```python
from build123d import *

# Parameters (mm, degrees)
SZKIC1_W                         = 100
SZKIC1_H                         = 28
OGOLNY_KSZTALT_DEPTH             = 50
ZAKRZYWUIENIE_OUTSIDE_W          = 53.052
ZAKRZYWUIENIE_OUTSIDE_H          = 75.052
WYCIECIE_KSZTAL_PRZOD_DEPTH      = 105
WYCIECIE_KSZTALTU_TYL_DEPTH      = 23
WYCIECIE_KSZTALTU_TYL_DEPTH_BACK = 99.5
SZKIC4_W                         = 30.5
SZKIC4_H                         = 10
SZKIC5_W                         = 39
SZKIC5_H                         = 10
PODBICIE_TYL_SPOD_DEPTH          = 5.5
SZKIC6_W                         = 100
SZKIC6_H                         = 8
PODBICIE_SRODEK_SPOD_DEPTH       = 4
PRZYCIECIE_OD_GORY_DEPTH         = 40
OTWORY_NA_SRUBY_DEPTH            = 90
OTWORY_NA_SRUBY_DEPTH_BACK       = 71
SZKIC8_R                         = 1.25
SZKIC9_W                         = 9
SZKIC9_H                         = 10
KTIR_KABLE_DEPTH                 = 10
WYTNIJ_WYCI_GNI_CIE3_DEPTH       = 84
WYTNIJ_WYCI_GNI_CIE3_DEPTH_BACK  = 81
SZKIC10_W                        = 29
SZKIC10_H                        = 10
WYTNIJ_WYCI_GNI_CIE4_DEPTH       = 59
WYTNIJ_WYCI_GNI_CIE4_DEPTH_BACK  = 55
SZKIC11_W                        = 10
SZKIC11_H                        = 15
SZKIC11_W_2                      = 17


with BuildPart() as part:
    # Szkic1 → ogolny ksztalt (new body)
    with BuildSketch(Plane(origin=(0, 0, 0), x_dir=(1, 0, 0), z_dir=(0, 1, 0))):
        with Locations((-50, 14)):
            Rectangle(SZKIC1_W, SZKIC1_H)
    extrude(amount=OGOLNY_KSZTALT_DEPTH)

    # zakrzywuienie outside → wyciecie ksztal przod (cut)
    with BuildSketch(Plane(origin=(0, 0, 0), x_dir=(0, 0, -1), z_dir=(1, 0, 0))):
        with Locations((14, 25)):
            Rectangle(ZAKRZYWUIENIE_OUTSIDE_W, ZAKRZYWUIENIE_OUTSIDE_H)
        with BuildLine():
            Line((28, 0), (18, 0))
            Line((18, 0), (0, 0))
            Line((0, 0), (0, 50))
            Line((0, 50), (18, 50))
            add(Edge.make_bspline(
                [(18, 50), (14.693585387, 12.992576306), (20.397077092, 0.692779903), (28, 0)],
                knots=[0, 0, 0, 0, 1, 1, 1, 1], degree=3))
        make_face(mode=Mode.SUBTRACT)
    extrude(amount=-WYCIECIE_KSZTAL_PRZOD_DEPTH, mode=Mode.SUBTRACT)

    # Szkic4 → wyciecie ksztaltu tyl (cut, two sides: drawn at the far end of the back side and taken through both)
    with BuildSketch(Plane(origin=(0, 0, 0), x_dir=(-1, 0, 0), z_dir=(0, -1, 0)).offset(-WYCIECIE_KSZTALTU_TYL_DEPTH_BACK)):
        with Locations((84.75, 5)):
            Rectangle(SZKIC4_W, SZKIC4_H)
        with Locations((15.25, 5)):
            Rectangle(SZKIC4_W, SZKIC4_H)
    extrude(amount=WYCIECIE_KSZTALTU_TYL_DEPTH + WYCIECIE_KSZTALTU_TYL_DEPTH_BACK, mode=Mode.SUBTRACT)

    # Szkic5 → podbicie tyl(spod) (cut)
    with BuildSketch(Plane(origin=(0, 0, 0), x_dir=(-1, 0, 0), z_dir=(0, -1, 0))):
        with Locations((50, 5)):
            Rectangle(SZKIC5_W, SZKIC5_H)
    extrude(amount=-PODBICIE_TYL_SPOD_DEPTH, mode=Mode.SUBTRACT)

    # Szkic6 → podbicie srodek(spod) (cut)
    with BuildSketch(Plane(origin=(0, 0, 0), x_dir=(-1, 0, 0), z_dir=(0, -1, 0))):
        with Locations((50, 14)):
            Rectangle(SZKIC6_W, SZKIC6_H)
    extrude(amount=-PODBICIE_SRODEK_SPOD_DEPTH, mode=Mode.SUBTRACT)

    # Szkic7 → przyciecie od gory (cut)
    with BuildSketch(Plane(origin=(0, 50, 0), x_dir=(1, 0, 0), z_dir=(0, 1, 0))):
        Polygon((0, 10), (-30.5, 10), (-30.5, 0), (-69.5, 0), (-69.5, 10), (-100, 10), (-100, 16), (0, 16), align=None)
    extrude(amount=-PRZYCIECIE_OD_GORY_DEPTH, mode=Mode.SUBTRACT)

    # Szkic8 → otwory na sruby (cut, two sides: drawn at the far end of the back side and taken through both)
    with BuildSketch(Plane(origin=(0, 5.5, 0), x_dir=(-1, 0, 0), z_dir=(0, -1, 0)).offset(-OTWORY_NA_SRUBY_DEPTH_BACK)):
        with Locations(Location((67, 4, 0), (0, 0, 270))):
            Circle(SZKIC8_R)
        with Locations(Location((33, 4, 0), (0, 0, 270))):
            Circle(SZKIC8_R)
        with Locations(Location((67.5, 14.5, 0), (0, 0, 270))):
            Circle(SZKIC8_R)
        with Locations(Location((32.5, 14.5, 0), (0, 0, 270))):
            Circle(SZKIC8_R)
        with Locations(Location((95, 14.5, 0), (0, 0, 270))):
            Circle(SZKIC8_R)
        with Locations(Location((5, 14.5, 0), (0, 0, 270))):
            Circle(SZKIC8_R)
    extrude(amount=OTWORY_NA_SRUBY_DEPTH + OTWORY_NA_SRUBY_DEPTH_BACK, mode=Mode.SUBTRACT)

    # Szkic9 → ktir kable (cut)
    with BuildSketch(Plane(origin=(0, 0, 0), x_dir=(-1, 0, 0), z_dir=(0, -1, 0))):
        with Locations((50, 13)):
            Rectangle(SZKIC9_W, SZKIC9_H)
        with Locations((14.5, 13)):
            Rectangle(SZKIC9_W, SZKIC9_H)
        with Locations((85.5, 13)):
            Rectangle(SZKIC9_W, SZKIC9_H)
    extrude(amount=-KTIR_KABLE_DEPTH, mode=Mode.SUBTRACT)

    # Szkic10 → Wytnij-wyciągnięcie3 (cut, two sides: drawn at the far end of the back side and taken through both)
    with BuildSketch(Plane.XZ.offset(-5.5).offset(-WYTNIJ_WYCI_GNI_CIE3_DEPTH_BACK)):
        with Locations((-50, -5)):
            Rectangle(SZKIC10_W, SZKIC10_H)
    extrude(amount=WYTNIJ_WYCI_GNI_CIE3_DEPTH + WYTNIJ_WYCI_GNI_CIE3_DEPTH_BACK, mode=Mode.SUBTRACT)

    # Szkic11 → Wytnij-wyciągnięcie4 (cut, two sides: drawn at the far end of the back side and taken through both)
    with BuildSketch(Plane.XY.offset(-16).offset(-WYTNIJ_WYCI_GNI_CIE4_DEPTH_BACK)):
        with Locations((-63.5, 17.5)):
            Rectangle(SZKIC11_W, SZKIC11_H)
        with Locations((-36.5, 17.5)):
            Rectangle(SZKIC11_W, SZKIC11_H)
        with Locations((-86, 17.5)):
            Rectangle(SZKIC11_W_2, SZKIC11_H)
        with Locations((-14, 17.5)):
            Rectangle(SZKIC11_W_2, SZKIC11_H)
    extrude(amount=WYTNIJ_WYCI_GNI_CIE4_DEPTH + WYTNIJ_WYCI_GNI_CIE4_DEPTH_BACK, mode=Mode.SUBTRACT)


solid = part.part
```
Part model, mm, in its own coordinate system. A direction names the side the tool comes from. Round coordinates to 2 decimals unless told otherwise and drop trailing zeros. Loops run counter-clockwise (first coordinate to the right, second up) from the corner with the lowest first, then second, coordinate; pieces in that order, holes last.
1. Two-plate mould, pull along X, no slides. Class faces 1 (the face through (-31.5, 16, -17)), 2 (the face through (-90, 7, -14)), 3 (the face through (-33, 5.5, -6)), 4 (the face through (-100, 16, -17)): pulls with the +X half, pulls with the -X half, needs draft (parallel to the pull), parting line crosses it, or undercut.
Solutions:
face 1: undercut
face 2: undercut
face 3: needs draft
face 4: pulls with the -X half
2. Slice it at A-A (z = -12.25). Give the cut face in (x, y), and give its area (3 significant figures).
Solutions:
outline: (-100, 4) - (-90, 4) - (-90, 10) - (-100, 10) - close; (-81, 4) - (-54.5, 4) - (-54.5, 10) - (-81, 10) - close; (-45.5, 4) - (-19, 4) - (-19, 10) - (-45.5, 10) - close; (-10, 4) - (0, 4) - (0, 10) - (-10, 10) - close
area: 438 mm2
3. Flat gauge pins, fed straight in: pin 1 (12 mm diameter, centred on x = -81, y = 13, fed in from +Z); pin 2 (2 mm diameter, centred on x = -67, z = -4, fed in from +Y); pin 3 (4 mm diameter, centred on x = -67, z = -5.5, fed in from -Y); pin 4 (1.3 mm diameter, centred on y = 7.5, z = -4, fed in from -X). Where does each tip first touch, or does it go through?
Solutions:
pin 1: stops at z = -10
pin 2: passes through
pin 3: stops at y = 5.5
pin 4: stops at x = -69.5
4. Drill centre lines: line 1 along X through (y, z) = (6.5, -1.5); line 2 along X through (y, z) = (20, -17.25); line 3 along Z through (x, y) = (-67, 6). Where is each one in solid material? Low to high.
Solutions:
line 1: x = -69.5 to -64.5, -35.5 to -30.5
line 2: x = -100 to -94.5, -77.5 to -68.5, -58.5 to -41.5, -31.5 to -22.5, -5.5 to 0
line 3: z = -20.8 to -15.65, -13.35 to -5.25, -2.75 to 0
5. Slice it at B-B (z = -7). Give the cut face in (x, y), and give its area (3 significant figures).
Solutions:
outline: (-69.5, 5.5) - (-64.5, 5.5) - (-64.5, 10) - (-69.5, 10) - close; (-35.5, 5.5) - (-30.5, 5.5) - (-30.5, 10) - (-35.5, 10) - close
area: 45.0 mm2
6. Slice it at C-C (y = 15.5). Count the separate pieces of the cut face and the enclosed holes in it, and give its area (3 significant figures).
Solutions:
separate pieces: 5
enclosed holes: 0
area: 95.3 mm2
7. 3-axis set-ups, long thin cutter, end or side, ignore diameter. For faces 5 (the face through (-5, 4, -13)), 6 (the face through (-5.5, 16, -17)), 7 (the face through (-5, 7, -10)), 8 (the face through (-50, 10, -17)): which of +Z, -Z, +X, -X, +Y, -Y reach the whole face in a straight line?
Solutions:
face 5: +Z, +X, -X, -Y
face 6: +Z, -Z
face 7: +Z, +X, +Y, -Y
face 8: +Z, -Y
